from build123d import *

# Parameters (mm, degrees)
F0_W     = 25.4
F0_H     = 25.4
F0_W_2   = 19.05
F0_H_2   = 19.05
F1_DEPTH = 609.6
F2_R     = 1.5875
F3_R     = 9.525
F4_DEPTH = 6.35
F5_R     = 3.175
F6_DEPTH = 25.4


with BuildPart() as f1:
    # F0 (on Right) → F1 (new body)
    with BuildSketch(Plane.YZ):
        with Locations((12.7, -12.7)):
            Rectangle(F0_W, F0_H)
        with Locations((12.7, -12.7)):
            Rectangle(F0_W_2, F0_H_2, mode=Mode.SUBTRACT)
    extrude(amount=F1_DEPTH)

    # F2
    f2_edges = [f1.edges().sort_by_distance(p)[0] for p in [
        (304.8, 0, 0),
        (304.8, 25.4, 0),
        (304.8, 0, -25.4),
        (304.8, 25.4, -25.4),
    ]]
    fillet(f2_edges, radius=F2_R)

    # F3 (on face) → F4 (cut)
    with BuildSketch(Plane.XY):
        with Locations((304.8, 12.7)):
            Circle(F3_R)
    extrude(amount=-F4_DEPTH, mode=Mode.SUBTRACT)

    # F5 (on face) → F6 (cut)
    with BuildSketch(Plane.XY):
        with Locations((304.8, 12.7)):
            Circle(F5_R)
    extrude(amount=-F6_DEPTH, mode=Mode.SUBTRACT)


solid = f1.part
Can you work these out from the model? Positions are in its coordinate system, mm. A direction names the side the tool comes from. Give positions to 0.01 mm unless a question says otherwise; leave off trailing zeros. Write each loop counter-clockwise with the first axis right and the second up, starting at its lowest first coordinate (ties: lowest second). Pieces come first, ordered by that corner, then holes. Notation, with made-up numbers: (77.25, 21) -> (94.25, 21) arc R23 ccw to (94.25, 46) -> close; hole circle Ø2 at (-9.75, 89). An arc over 180 degrees is marked (long way). Answer as a JSON object with one key per item and string values. Group by question number.
Item 1: I'm going to push a flat-ended pin straight in: P1, Ø5, axis at x = 304.8, y = 12.7, coming from the -Z side. Where does the tip first touch, or does it pass through?
Item 2: For faces 1 (the face through (301, 13, -25.4)), 2 (the face through (150, 13, -3.175)), which set-ups out of +Z, -Z, +X, -X, +Y, -Y let a thin tool reach every point of the face, with its end or its side?
Item 3: Suppose I cut it at B-B (z = -14.25). Please give me the cut outline in (x, y) (3 decimals).
Item 4: Suppose I cut it at A-A (x = 164.5). Please give me the cut outline in (y, z) (1 decimal), plus the area to 3 significant figures.
Item 5: Please list where these lines run through material, in increasing order: line 1 (Y direction, x = 187, z = -16) (3 decimals); line 2 (X direction, y = 12.7, z = -1.5) (3 decimals); line 3 (Z direction, x = 522, y = 10.25) (3 decimals). Write a range as [from, to].
Item 6: We'd pull the mould along X, two halves only. Please class faces 3 (the face through (295.284, 13.119, -1.565)), 4 (the face through (301, 22.225, -13)), 5 (the face through (0, 13, -24)), 6 (the face through (609.6, 13, -24)): +X half, -X half, draft (parallel to the pull), parting line (faces both ways), or undercut.
Findings:
{
 "1": {"P1": "passes through"},
 "2": {"face 1": "-Z, +X, -X, +Y, -Y", "face 2": "+X, -X"},
 "3": {"outline": "(0, 0) -> (609.6, 0) -> (609.6, 3.175) -> (0, 3.175) -> close; (0, 22.225) -> (609.6, 22.225) -> (609.6, 25.4) -> (0, 25.4) -> close"},
 "4": {"outline": "(0, -23.8) arc R1.6 ccw to (1.6, -25.4) -> (23.8, -25.4) arc R1.6 ccw to (25.4, -23.8) -> (25.4, -1.6) arc R1.6 ccw to (23.8, 0) -> (1.6, 0) arc R1.6 ccw to (0, -1.6) -> close; hole (3.2, -22.2) -> (22.2, -22.2) -> (22.2, -3.2) -> (3.2, -3.2) -> close", "area": "280 mm²"},
 "5": {"line 1": "y = [0, 3.175], [22.225, 25.4]", "line 2": "x = [0, 295.275], [314.325, 609.6]", "line 3": "z = [-25.4, -22.225], [-3.175, 0]"},
 "6": {"face 3": "undercut", "face 4": "draft", "face 5": "-X half", "face 6": "+X half"}
}
